CAD build for the part. Positions are in the model's coordinates, mm. A direction names the side the tool comes from. Round coordinates to 2 decimals unless told otherwise and drop trailing zeros. Write each loop counter-clockwise with the first axis right and the second up, starting at its lowest first coordinate (ties: lowest second). Pieces come first, ordered by that corner, then holes. Notation, with made-up numbers: (55, 68) -> (103, 68) arc R33 ccw to (103, 96) -> close; hole circle Ø8 at (8, 8). An arc over 180 degrees is marked (long way). Put each result on its own line as item: value. Start each with the question number.
1. Saw through at B-B on y = 27.5. List the corners of the cut face in (x, z) (3 decimals), and give its area (3 significant figures).
2. 3-axis set-ups, long thin cutter, end or side, ignore diameter. For faces 5 (the flat face through (13, 3.175, 257)), 6 (the flat face through (9, 57.15, 257)), 7 (the cylindrical face through (11.842, 1.565, 215.278)): which of +Z, -Z, +X, -X, +Y, -Y reach the whole face in a straight line?
3. Saw through at A-A on z = 420. List the corners of the cut face in (x, y) (3 decimals).
4. Flat gauge pins, fed straight in: P1, Ø2.5, axis at y = 2, z = 325, coming from the +X side; P2, Ø3.5, axis at y = 55.5, z = 414.5, coming from the +X side (3 decimals); P3, Ø12, axis at y = 37.5, z = 414, coming from the +X side (3 decimals). Where does each tip first touch, or does it go through?
5. Pull direction Y, two halves, no side cores. Call faces 1 (the flat face through (11, 0, 257)), 2 (the flat face through (3, 33, 0)), 3 (the flat face through (11, 53.975, 257)), 4 (the flat face through (3.175, 29, 257)): pulls with the +Y half, pulls with the -Y half, needs draft (parallel to the pull), parting line crosses it, or undercut.
6. Drill centre lines: line 1 (Y direction, x = 4.5, z = 360.5) (3 decimals); line 2 (X direction, y = 3.5, z = 194) (3 decimals); line 3 (Y direction, x = 20.5, z = 340) (3 decimals). Where is each one in solid material? Low to high. Write a range as from..to.
Autodesk Inventor part; units mm, degrees
ref_plane "YZ Plane" through (0, 0, 0) normal (1, 0, 0) x (0, 1, 0)
ref_plane "XZ Plane" through (0, 0, 0) normal (0, 1, 0) x (-1, 0, 0)
ref_plane "XY Plane" through (0, 0, 0) normal (0, 0, 1) x (1, 0, 0)
sketch "Sketch1" plane through (0, 0, 0) normal (0, 0, 1) x (1, 0, 0)
  line L0 (0, 0) -> (22.225, 0)
  line L1 (22.225, 0) -> (22.225, 57.15)
  line L2 (22.225, 57.15) -> (0, 57.15)
  line L3 (0, 57.15) -> (0, 0)
  line L4 (3.175, 3.175) -> (22.225, 3.175)
  line L5 (22.225, 3.175) -> (22.225, 53.975)
  line L6 (22.225, 53.975) -> (3.175, 53.975)
  line L7 (3.175, 53.975) -> (3.175, 3.175)
  dimension "d0" = 3.175
  dimension "d1" = 3.175
  dimension "d2" = 3.175
  dimension "d3" = 57.15
  dimension "d4" = 22.225
extrude "Extrusion1" add sketch "Sketch1" along normal blind 520.7 contours L3 L2 L1 L6 L7 L4 L0
sketch "Sketch2" plane through (0, 57.15, 0) normal (0, 1, 0) x (1, 0, 0)
  line L0 (22.225, 0) -> (22.225, -520.7)
  line L1 (0, 0) -> (0, -520.7)
  line L2 (22.7547, 0) -> (0, 0)
  line L3 (22.225, -85.725) -> (15.875, -85.725)
  line L4 (15.875, -85.725) -> (15.875, -155.575)
  line L5 (15.875, -155.575) -> (22.225, -155.575)
  line L6 (22.225, -155.575) -> (22.225, -85.725)
  line L7 (22.225, -180.975) -> (11.43, -180.975)
  line L8 (11.43, -180.975) -> (11.43, -206.375)
  line L9 (11.43, -206.375) -> (22.225, -206.375)
  line L10 (22.225, -206.375) -> (22.225, -180.975)
  arc A0 (22.225, -21.2995) -> (22.225, -54.9005) centre (41.275, -38.1) ccw
  circle A1 centre (12.7, -9.525) radius 3.175
  circle A2 centre (12.7, -228.6) radius 3.175
  line L11 (3.175, 0) -> (3.175, -520.7)
  line L12 (22.225, 0) -> (0, 0)
  line L13 (22.225, -21.2995) -> (22.225, -54.9005)
  line L14 (0, -260.35) -> (22.225, -260.35) construction
  line L15 (22.225, -339.725) -> (11.43, -339.725)
  line L16 (11.43, -339.725) -> (11.43, -314.325)
  line L17 (22.225, -314.325) -> (22.225, -339.725)
  line L18 (11.43, -314.325) -> (22.225, -314.325)
  circle A3 centre (12.7, -292.1) radius 3.175
  line L19 (15.875, -365.125) -> (22.225, -365.125)
  line L20 (15.875, -434.975) -> (15.875, -365.125)
  line L21 (22.225, -365.125) -> (22.225, -434.975)
  line L22 (22.225, -434.975) -> (15.875, -434.975)
  arc A4 (22.225, -465.7995) -> (22.225, -499.4005) centre (41.275, -482.6) ccw
  circle A5 centre (12.7, -511.175) radius 3.175
  line L23 (22.225, -520.7) -> (0, -520.7)
  line L24 (22.225, -499.4005) -> (22.225, -465.7995)
  dimension "d7" = 85.725
  dimension "d8" = 69.85
  dimension "d9" = 6.35
  dimension "d10" = 180.975
  dimension "d11" = 25.4
  dimension "d12" = 25.4
  dimension "d13" = 38.1
  dimension "d14" = 9.525
  dimension "d15" = 6.35
  dimension "d16" = 228.6
  dimension "d17" = 38.1
  dimension "d18" = 11.43
  dimension "d21" = 260.35
extrude "Extrusion2" cut sketch "Sketch2" against normal blind 3.175 contours L0 A0 | L0 L5 L4 L3 | A4 L0 | L0 L9 L8 L7 | L22 L20 L19 L0 | L0 L15 L16 L18 | A1 | A2 | A3 | A5
sketch "Sketch3" plane through (0, 0, 0) normal (0, -1, 0) x (1, 0, 0)
  line L0 (0, 0) -> (0, 520.7)
  line L1 (0, 0) -> (22.225, 0)
  line L2 (22.225, 0) -> (22.225, 520.7)
  line L3 (0, 0) -> (0, 301.9932)
  line L4 (0, 0) -> (22.225, 0)
  line L5 (22.225, 0) -> (22.225, 21.2995)
  arc A0 (7.9375, 187.325) -> (22.225, 160.8085) centre (39.6875, 187.325) ccw
  line L6 (7.9375, 187.325) -> (7.9375, 200.025)
  arc A1 (22.225, 226.5415) -> (7.9375, 200.025) centre (39.6875, 200.025) ccw
  arc A2 (22.225, 54.9005) -> (22.225, 21.2995) centre (41.275, 38.1) ccw
  circle A3 centre (12.7, 9.525) radius 3.175
  circle A4 centre (12.7, 228.6) radius 3.175
  line L7 (3.175, 0) -> (3.175, 520.7)
  line L8 (0, 260.35) -> (22.225, 260.35) construction
  line L9 (22.225, 160.8085) -> (22.225, 226.5415)
  line L10 (22.225, 226.5415) -> (22.225, 302.1048)
  line L11 (22.225, 21.2995) -> (22.225, 54.9005)
  line L12 (22.225, 54.9005) -> (22.225, 160.8085)
  arc A5 (22.225, 359.8915) -> (7.9375, 333.375) centre (39.6875, 333.375) ccw
  line L13 (7.9375, 333.375) -> (7.9375, 320.675)
  arc A6 (7.9375, 320.675) -> (22.225, 294.1585) centre (39.6875, 320.675) ccw
  arc A7 (22.225, 499.4005) -> (22.225, 465.7995) centre (41.275, 482.6) ccw
  circle A8 centre (12.7, 511.175) radius 3.175
  circle A9 centre (12.7, 292.1) radius 3.175
  line L14 (22.225, 359.8915) -> (22.225, 294.1585)
  line L15 (22.225, 499.4005) -> (22.225, 465.7995)
  dimension "d22" = 31.75
  dimension "d23" = 12.7
  dimension "d24" = 187.325
  dimension "d25" = 7.9375
  dimension "d26" = 38.1
  dimension "d27" = 38.1
  dimension "d28" = 25.4
  dimension "d29" = 260.35
extrude "Extrusion3" cut sketch "Sketch3" against normal blind 3.175
fillet "Fillet1" radius 3.175 8 edges at (15.875, 55.5625, 434.975) (15.875, 55.5625, 365.125) (11.43, 55.5625, 339.725) (11.43, 55.5625, 314.325) (11.43, 55.5625, 206.375) (11.43, 55.5625, 180.975) (15.875, 55.5625, 155.575) (15.875, 55.5625, 85.725)
equation "\"d1\" = d0"
equation "\"d2\" = d0"
properties part number "2.25 U frame 2"
Return value:
1. outline: (0, 0) -> (3.175, 0) -> (3.175, 520.7) -> (0, 520.7) -> close
1. area: 1,650 mm^2
2. face 5: +Z, -Z, +X
2. face 6: +Z, -Z, +X, -X, +Y
2. face 7: +X, -Y
3. outline: (0, 0) -> (22.225, 0) -> (22.225, 3.175) -> (3.175, 3.175) -> (3.175, 53.975) -> (15.875, 53.975) -> (15.875, 57.15) -> (0, 57.15) -> close
4. P1: stops at x = 7.94
4. P2: stops at x = 15.875
4. P3: stops at x = 3.175
5. face 1: pulls with the -Y half
5. face 2: needs draft
5. face 3: undercut
5. face 4: undercut
6. line 1: y = 0..3.175, 53.975..57.15
6. line 2: x = 0..3.175
6. line 3: y = 53.975..57.15
